from build123d import *

# Parameters (mm, degrees)
BOSS_EXTRUDE1_DEPTH     = 3
SKETCH2_R               = 3.575
CUT_EXTRUDE1_DEPTH      = 3.95
BOSS_EXTRUDE2_DEPTH     = 1.64
SKETCH4_R               = 3.25
CUT_EXTRUDE2_DEPTH      = 63.566201739
CAVITY1_OUTLINE_R       = 3.25
CAVITY1_DEPTH           = 4.64
CAVITY1_START           = 3.19
CAVITY1_2_DEPTH         = 1.45
CUT_EXTRUDE4_DEPTH      = 63.566201739
BOSS_EXTRUDE3_START     = -4.64
BOSS_EXTRUDE3_DEPTH     = 4.64
BOSS_EXTRUDE4_DEPTH     = 4.64
BOSS_EXTRUDE5_DEPTH     = 4.64
CUT_EXTRUDE5_DEPTH      = 1.45
SKETCH7_R               = 1
CUT_EXTRUDE6_DEPTH      = 4.64
CUT_EXTRUDE7_DEPTH      = 68.226628653
CUT_EXTRUDE7_DEPTH_BACK = 68.226628653
SKETCH10_W              = 23.28963149
SKETCH10_H              = 12.3
SKETCH10_W_2            = 22.98963149
SKETCH10_H_2            = 12
CUT_EXTRUDE8_DEPTH      = 1.45
CUT_EXTRUDE9_DEPTH      = 1.45
SKETCH14_W              = 12.3
SKETCH14_H              = 3.19
CUT_EXTRUDE10_DEPTH     = 1
SKETCH15_W              = 12.3
SKETCH15_H              = 3.19
CUT_EXTRUDE11_DEPTH     = 1
CUT_EXTRUDE12_DEPTH     = 1
CUT_EXTRUDE13_DEPTH     = 1


# Read off the part's stored shape, not the designer's step: Cavity1
with BuildPart() as part:
    # Sketch1 → Boss-Extrude1 (new body)
    with BuildSketch(Plane(origin=(0, 0, 0), x_dir=(1, 0, 0), z_dir=(0, 1, 0))):
        with BuildLine():
            Line((0, 7), (55, 7))
            ThreePointArc((55, 7), (62, 0), (55, -7))
            Line((55, -7), (0, -7))
            ThreePointArc((0, -7), (-7, 0), (0, 7))
        make_face()
    extrude(amount=BOSS_EXTRUDE1_DEPTH)

    # Sketch2 → Cut-Extrude1 (cut)
    with BuildSketch(Plane.XZ):
        with Locations(Location((0, 0, 0), (0, 0, 270))):
            Circle(SKETCH2_R)
    extrude(amount=-CUT_EXTRUDE1_DEPTH, mode=Mode.SUBTRACT)

    # Sketch3 → Boss-Extrude2 (add)
    with BuildSketch(Plane(origin=(0, 3, 0), x_dir=(1, 0, 0), z_dir=(0, 1, 0))):
        with BuildLine():
            Line((0, -7), (55, -7))
            ThreePointArc((55, -7), (62, 0), (55, 7))
            Line((55, 7), (0, 7))
            ThreePointArc((0, 7), (-7, 0), (0, -7))
        make_face()
        with BuildLine():
            Line((14.43004688, 2.119993993), (2.468524523, 2.816276208))
            ThreePointArc((2.468524523, 2.816276208), (-3.745, 0), (2.468524523, -2.816276208))
            Line((2.468524523, -2.816276208), (14.43004688, -2.119993993))
            ThreePointArc((14.43004688, -2.119993993), (16.545, 0), (14.43004688, 2.119993993))
        make_face(mode=Mode.SUBTRACT)
    extrude(amount=BOSS_EXTRUDE2_DEPTH)

    # Sketch4 → Cut-Extrude2 (cut, through all)
    with BuildSketch(Plane(origin=(0, 4.64, 0), x_dir=(1, 0, 0), z_dir=(0, 1, 0))):
        with Locations(Location((55, 0, 0), (0, 0, 270))):
            Circle(SKETCH4_R)
    extrude(amount=-CUT_EXTRUDE2_DEPTH, mode=Mode.SUBTRACT)

    # Cavity1 outline → Cavity1 (cut)
    with BuildSketch(Plane(origin=(0, 0, 0), x_dir=(1, 0, 0), z_dir=(0, 1, 0))):
        with BuildLine():
            Line((58.605551275, 6), (38, 6))
            Line((38, 6), (38, -6))
            Line((38, -6), (58.605551275, -6))
            ThreePointArc((58.605551275, -6), (59.949747468, -4.949747468), (61, -3.605551275))
            Line((61, -3.605551275), (61, 3.605551275))
            ThreePointArc((61, 3.605551275), (59.949747468, 4.949747468), (58.605551275, 6))
        make_face()
        with Locations((55, 0)):
            Circle(CAVITY1_OUTLINE_R, mode=Mode.SUBTRACT)
    extrude(amount=CAVITY1_DEPTH, mode=Mode.SUBTRACT)

    # Cavity1 2 outline → Cavity1 2 (cut)
    with BuildSketch(Plane(origin=(0, 0, 0), x_dir=(1, 0, 0), z_dir=(0, 1, 0)).offset(CAVITY1_START)):
        with BuildLine():
            Line((33.3, 0.5), (34.605619966, 0.5))
            ThreePointArc((34.605619966, 0.5), (36.47164537, 0), (34.605619966, -0.5))
            Line((34.605619966, -0.5), (33.3, -0.5))
            Line((33.3, -0.5), (33.3, -6))
            Line((33.3, -6), (38, -6))
            Line((38, -6), (38, 6))
            Line((38, 6), (33.3, 6))
            Line((33.3, 6), (33.3, 0.5))
        make_face()
        with BuildLine():
            ThreePointArc((61, -3.605551275), (62, 0), (61, 3.605551275))
            Line((61, 3.605551275), (61, -3.605551275))
        make_face()
    extrude(amount=CAVITY1_2_DEPTH, mode=Mode.SUBTRACT)

    # Sketch5 → Cut-Extrude4 (cut, through all)
    with BuildSketch(Plane.XZ):
        with BuildLine():
            Line((61, 3.605551275), (61, -3.605551275))
            ThreePointArc((61, -3.605551275), (62, 0), (61, 3.605551275))
        make_face()
    extrude(amount=-CUT_EXTRUDE4_DEPTH, mode=Mode.SUBTRACT)

    # Sketch6 → Boss-Extrude3 (add)
    with BuildSketch(Plane(origin=(0, 4.64, 0), x_dir=(1, 0, 0), z_dir=(0, 1, 0)).offset(BOSS_EXTRUDE3_START)):
        with BuildLine():
            Line((61, -6), (58.605551275, -6))
            ThreePointArc((58.605551275, -6), (56.870828693, -6.745368782), (55, -7))
            Line((55, -7), (66.7, -7))
            Line((66.7, -7), (66.7, 7))
            Line((66.7, 7), (55, 7))
            ThreePointArc((55, 7), (56.870828693, 6.745368782), (58.605551275, 6))
            Line((58.605551275, 6), (61, 6))
            Line((61, 6), (65.7, 6))
            Line((65.7, 6), (65.7, 0.5))
            Line((65.7, 0.5), (65.7, -0.5))
            Line((65.7, -0.5), (65.7, -6))
            Line((65.7, -6), (61, -6))
        make_face()
        with BuildLine():
            Line((58.605551275, -6), (33.3, -6))
            Line((33.3, -6), (33.3, -7))
            Line((33.3, -7), (55, -7))
            ThreePointArc((55, -7), (56.870828693, -6.745368782), (58.605551275, -6))
        make_face()
        with BuildLine():
            Line((33.3, 7), (33.3, 6))
            Line((33.3, 6), (58.605551275, 6))
            ThreePointArc((58.605551275, 6), (56.870828693, 6.745368782), (55, 7))
            Line((55, 7), (33.3, 7))
        make_face()
    extrude(amount=BOSS_EXTRUDE3_DEPTH)

    # Sketch6<3> → Boss-Extrude4 (add)
    with BuildSketch(Plane(origin=(0, 4.64, 0), x_dir=(1, 0, 0), z_dir=(0, 1, 0))):
        with BuildLine():
            Line((64.394380034, -0.5), (65.7, -0.5))
            Line((65.7, -0.5), (65.7, 0.5))
            Line((65.7, 0.5), (64.394380034, 0.5))
            ThreePointArc((64.394380034, 0.5), (62.52835463, 0), (64.394380034, -0.5))
        make_face()
    extrude(amount=-BOSS_EXTRUDE4_DEPTH)

    # Sketch6<5> → Boss-Extrude5 (add)
    with BuildSketch(Plane(origin=(0, 4.64, 0), x_dir=(1, 0, 0), z_dir=(0, 1, 0))):
        with BuildLine():
            Line((61, 6), (61, -6))
            Line((61, -6), (65.7, -6))
            Line((65.7, -6), (65.7, -0.5))
            Line((65.7, -0.5), (64.394380034, -0.5))
            ThreePointArc((64.394380034, -0.5), (62.52835463, 0), (64.394380034, 0.5))
            Line((64.394380034, 0.5), (65.7, 0.5))
            Line((65.7, 0.5), (65.7, 6))
            Line((65.7, 6), (61, 6))
        make_face()
    extrude(amount=-BOSS_EXTRUDE5_DEPTH)

    # Sketch6<6> → Cut-Extrude5 (cut)
    with BuildSketch(Plane(origin=(0, 4.64, 0), x_dir=(1, 0, 0), z_dir=(0, 1, 0))):
        with BuildLine():
            Line((61, 6), (61, -6))
            Line((61, -6), (65.7, -6))
            Line((65.7, -6), (65.7, -0.5))
            Line((65.7, -0.5), (64.394380034, -0.5))
            ThreePointArc((64.394380034, -0.5), (62.52835463, 0), (64.394380034, 0.5))
            Line((64.394380034, 0.5), (65.7, 0.5))
            Line((65.7, 0.5), (65.7, 6))
            Line((65.7, 6), (61, 6))
        make_face()
    extrude(amount=-CUT_EXTRUDE5_DEPTH, mode=Mode.SUBTRACT)

    # Sketch7 → Cut-Extrude6 (cut)
    with BuildSketch(Plane(origin=(0, 4.64, 0), x_dir=(1, 0, 0), z_dir=(0, 1, 0))):
        with Locations(Location((63.52835463, 0, 0), (0, 0, 270))):
            Circle(SKETCH7_R)
        with Locations(Location((35.47164537, 0, 0), (0, 0, 270))):
            Circle(SKETCH7_R)
    extrude(amount=-CUT_EXTRUDE6_DEPTH, mode=Mode.SUBTRACT)

    # Sketch10 → Cut-Extrude7 (cut, two sides: drawn at the far end of the back side and taken through both)
    with BuildSketch(Plane.XZ.offset(-CUT_EXTRUDE7_DEPTH_BACK)):
        with Locations((49.494815745, 0)):
            Rectangle(SKETCH10_W, SKETCH10_H)
        with Locations((49.494815745, 0)):
            Rectangle(SKETCH10_W_2, SKETCH10_H_2, mode=Mode.SUBTRACT)
    extrude(amount=CUT_EXTRUDE7_DEPTH + CUT_EXTRUDE7_DEPTH_BACK, mode=Mode.SUBTRACT)

    # Sketch11 → Cut-Extrude8 (cut)
    with BuildSketch(Plane(origin=(0, 4.64, 0), x_dir=(1, 0, 0), z_dir=(0, 1, 0))):
        Polygon((37.85, -6), (33.3, -6), (33.3, -0.5), (33.15, -0.5), (33.15, -6.15), (37.85, -6.15), align=None)
        Polygon((33.3, 0.5), (33.3, 6), (37.85, 6), (37.85, 6.15), (33.15, 6.15), (33.15, 0.5), align=None)
    extrude(amount=-CUT_EXTRUDE8_DEPTH, mode=Mode.SUBTRACT)

    # Sketch13 → Cut-Extrude9 (cut)
    with BuildSketch(Plane(origin=(0, 4.64, 0), x_dir=(1, 0, 0), z_dir=(0, 1, 0))):
        Polygon((61.13963149, -6), (65.7, -6), (65.7, -0.5), (65.85, -0.5), (65.85, -6.15), (61.13963149, -6.15), align=None)
        Polygon((61.13963149, 6), (65.7, 6), (65.7, 0.5), (65.85, 0.5), (65.85, 6.15), (61.13963149, 6.15), align=None)
    extrude(amount=-CUT_EXTRUDE9_DEPTH, mode=Mode.SUBTRACT)

    # Sketch14 → Cut-Extrude10 (cut)
    with BuildSketch(Plane(origin=(37.85, 0, 0), x_dir=(0, 0, -1), z_dir=(1, 0, 0))):
        with Locations((0, 1.595)):
            Rectangle(SKETCH14_W, SKETCH14_H)
    extrude(amount=-CUT_EXTRUDE10_DEPTH, mode=Mode.SUBTRACT)

    # Sketch15 → Cut-Extrude11 (cut)
    with BuildSketch(Plane.ZY.offset(-61.13963149)):
        with Locations((0, 1.595)):
            Rectangle(SKETCH15_W, SKETCH15_H)
    extrude(amount=-CUT_EXTRUDE11_DEPTH, mode=Mode.SUBTRACT)

    # Sketch16 → Cut-Extrude12 (cut)
    with BuildSketch(Plane(origin=(0, 3.19, 0), x_dir=(1, 0, 0), z_dir=(0, 1, 0))):
        with BuildLine():
            Line((62.13963149, 6.15), (62.13963149, -6.15))
            Line((62.13963149, -6.15), (65.85, -6.15))
            Line((65.85, -6.15), (65.85, -0.5))
            Line((65.85, -0.5), (64.394380034, -0.5))
            ThreePointArc((64.394380034, -0.5), (62.52835463, 0), (64.394380034, 0.5))
            Line((64.394380034, 0.5), (65.85, 0.5))
            Line((65.85, 0.5), (65.85, 6.15))
            Line((65.85, 6.15), (62.13963149, 6.15))
        make_face()
    extrude(amount=-CUT_EXTRUDE12_DEPTH, mode=Mode.SUBTRACT)

    # Sketch17 → Cut-Extrude13 (cut)
    with BuildSketch(Plane(origin=(0, 3.19, 0), x_dir=(1, 0, 0), z_dir=(0, 1, 0))):
        with BuildLine():
            Line((36.85, -6.15), (36.85, 6.15))
            Line((36.85, 6.15), (33.15, 6.15))
            Line((33.15, 6.15), (33.15, 0.5))
            Line((33.15, 0.5), (34.605619966, 0.5))
            ThreePointArc((34.605619966, 0.5), (36.47164537, 0), (34.605619966, -0.5))
            Line((34.605619966, -0.5), (33.15, -0.5))
            Line((33.15, -0.5), (33.15, -6.15))
            Line((33.15, -6.15), (36.85, -6.15))
        make_face()
    extrude(amount=-CUT_EXTRUDE13_DEPTH, mode=Mode.SUBTRACT)


solid = part.part
For this review, take the finished solid that the model builds, in its own axes (mm). A direction names the side the tool comes from. Give positions to 0.01 mm unless a question says otherwise; leave off trailing zeros. Loops run counter-clockwise (first coordinate to the right, second up) from the corner with the lowest first, then second, coordinate; pieces in that order, holes last.
Item 1: Take a section at C-C, the plane y = 1.4. State the section outline as (x, z) points (3 decimals).
Item 2: Take a section at B-B, the plane x = 40. State the section outline as (y, z) points.
Item 3: Insertion check: pin 1 (8 mm diameter, centred on x = 6.5, z = -1, fed in from +Y); pin 2 (1.1 mm diameter, centred on x = 34.5, z = -1.5, fed in from +Y); pin 3 (2.5 mm diameter, centred on y = 3.5, z = -4, fed in from -X); pin 4 (2.5 mm diameter, centred on y = 1, z = -3, fed in from -X). Each pin has a flat end and moves straight along its axis. Give the tip position at first contact, or say it passes through.
Item 4: Draft analysis for pull direction Z (two halves, no side actions). For faces 3 (the flat face through (34, 2, -7)), 4 (the flat face through (21, 4.64, 0)), 5 (the flat face through (36.85, 1, 0)), state which applies: +Z half, -Z half, draft (parallel to the pull), parting line (faces both ways), or undercut.
Item 5: Tool access review of faces 1 (the flat face through (8.366, 3.809, 2.473)), 2 (the cylindrical face through (-7, 2, 0)): name each direction out of +Z, -Z, +X, -X, +Y, -Y from which nothing blocks a thin tool from reaching the whole face with its end or side.
Item 6: For line 1 along X through (y, z) = (2.3, 0) (3 decimals); line 2 along X through (y, z) = (4.15, 0) (3 decimals); line 3 along Z through (x, y) = (54, 1.55), list the stretches that pass through material, from the lowest coordinate up.
Item 7: Take a section at A-A, the plane z = -5. State the section outline as (x, y) points.
Item 8: Take a section at D-D, the plane x = 11.5. State the section outline as (y, z) points.
Calculated:
1. outline: (0, -7) - (66.7, -7) - (66.7, 7) - (0, 7) arc R7 ccw to start; hole circle Ø7.15 at (0, 0); hole circle Ø2 at (35.472, 0); hole (36.85, -6.15) - (62.14, -6.15) - (62.14, 6.15) - (36.85, 6.15) - close; hole circle Ø2 at (63.528, 0)
2. outline: (0, -7) - (4.64, -7) - (4.64, -6.15) - (0, -6.15) - close; (0, 6.15) - (4.64, 6.15) - (4.64, 7) - (0, 7) - close
3. pin 1: stops at y = 4.64
3. pin 2: stops at y = 2.19
3. pin 3: stops at x = -6.44
3. pin 4: stops at x = -6.78
4. face 3: -Z half
4. face 4: draft
4. face 5: undercut
5. face 1: +Y
5. face 2: -X, +Y, -Y
6. line 1: x = -7 to -3.575, 3.575 to 34.472, 64.528 to 66.7
6. line 2: x = -7 to -3.745, 16.545 to 34.472, 64.528 to 66.7
6. line 3: z = -7 to -6.15, 6.15 to 7
7. outline: (-4.9, 0) - (36.85, 0) - (36.85, 2.19) - (33.15, 2.19) - (33.15, 4.64) - (-4.9, 4.64) - close; (62.14, 0) - (66.7, 0) - (66.7, 4.64) - (65.85, 4.64) - (65.85, 2.19) - (62.14, 2.19) - close
8. outline: (0, -7) - (4.64, -7) - (4.64, -2.29) - (3, -2.29) - (3, 2.29) - (4.64, 2.29) - (4.64, 7) - (0, 7) - close
